The drawing under review shows one solid part. Ordinate dimensions are in mm from its lowest x, y, z. Give positions to 0.01 mm unless a question says otherwise; leave off trailing zeros. Write each loop counter-clockwise with the first axis right and the second up, starting at its lowest first coordinate (ties: lowest second). Pieces come first, ordered by that corner, then holes.
Q1. We need section B-B (y = 0.85). Write out the cut boundary in (x, z).
Q2. For line 1 (Z direction, x = 38, y = 1.9), list the stretches that pass through material, from the lowest coordinate up.
Q3. We need section A-A (x = 25.5). Write out the cut boundary in (y, z), then the cut area to 3 significant figures.
Q4. Insertion check: P1, Ø0.9, axis at x = 19.5, z = 80.5, coming from the +Y side; P2, Ø0.9, axis at x = 46.5, z = 80.5, coming from the -Y side; P3, Ø1.1, axis at x = 49, y = 1, coming from the +Z side. Each pin has a flat end and moves straight along its axis. Give the tip position at first contact, or say it passes through.
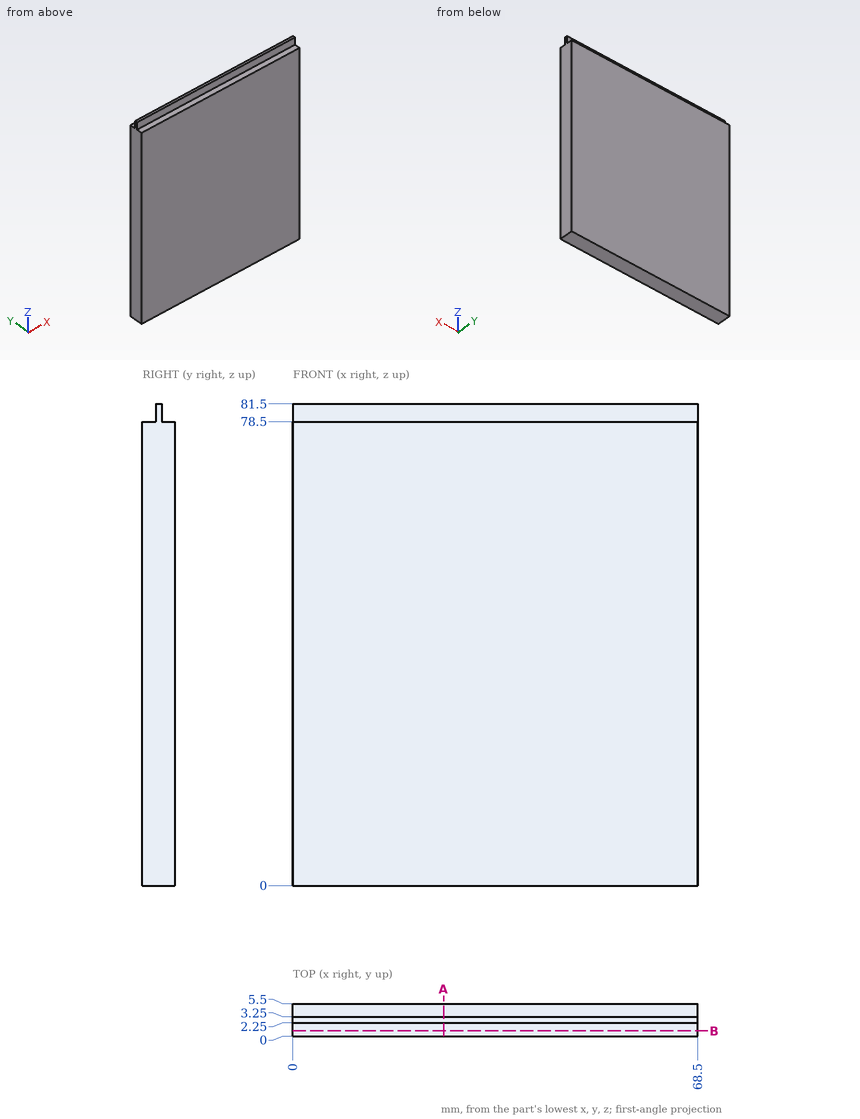
Computed:
1. outline: (0, 0) - (68.5, 0) - (68.5, 78.5) - (0, 78.5) - close
2. line 1: z = 0 to 78.5
3. outline: (0, 0) - (5.5, 0) - (5.5, 78.5) - (3.25, 78.5) - (3.25, 81.5) - (2.25, 81.5) - (2.25, 78.5) - (0, 78.5) - close
3. area: 435 mm2
4. P1: stops at y = 3.25
4. P2: stops at y = 2.25
4. P3: stops at z = 78.5
